from build123d import *

# Parameters (mm, degrees)
BOSS_EXTRUDE2_DEPTH = 3.175
FILLET3_R           = 7.62
FILLET4_R           = 5.08


with BuildPart() as part:
    # Sketch2 → Boss-Extrude2 (new body)
    with BuildSketch(Plane(origin=(0, 0, 0), x_dir=(1, 0, 0), z_dir=(0, 1, 0))):
        Polygon((444.5, 96.52), (0, 96.52), (57.15, 0), (444.5, 0), align=None)
    extrude(amount=BOSS_EXTRUDE2_DEPTH)

    # Fillet3
    fillet3_edges = [part.edges().sort_by_distance(p)[0] for p in [
        (57.15, 1.5875, 0),
        (444.5, 1.5875, -96.52),
        (444.5, 1.5875, 0),
    ]]
    fillet(fillet3_edges, radius=FILLET3_R)

    # Fillet4
    fillet4_edges = [part.edges().sort_by_distance(p)[0] for p in [
        (0, 1.5875, -96.52),
    ]]
    fillet(fillet4_edges, radius=FILLET4_R)


solid = part.part
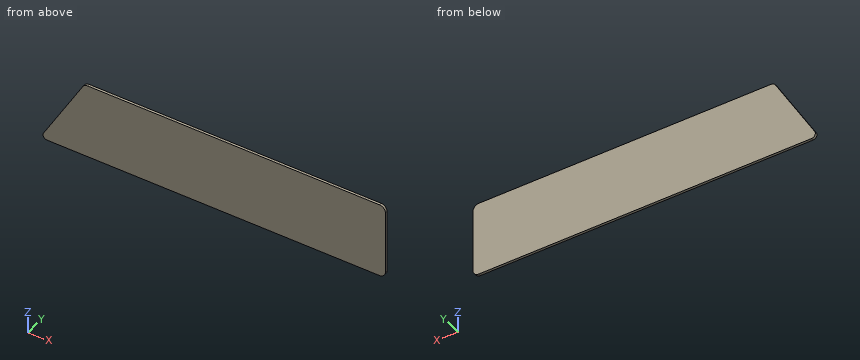
Source: CAD feature listing. Evaluate the final solid. Frame: model axes, mm. Coordinates: 2 decimals unless noted, no trailing zeros. Loops run counter-clockwise (first coordinate to the right, second up) from the corner with the lowest first, then second, coordinate; pieces in that order, holes last. Notation, with made-up numbers: (21.25, 10) - (68.25, 10) arc R17 cw to (68.25, 23) - close; hole circle Ø2 at (76.25, 66). An arc over 180 degrees is marked (long way). One line per question, with ' | ' between items.
1) Section C-C, the plane z = -45.5. Return loops of the section in (x, y) (3 decimals).
Report:
outline: (30.209, 0) - (444.5, 0) - (444.5, 3.175) - (30.209, 3.175) - close
2) Line query: line 1 along Z through (x, y) = (42.5, 0.8); line 2 along X through (y, z) = (0.8, -14.5); line 3 along X through (y, z) = (1.75, -70). Output: solid intervals per line, ascending.
Report:
line 1: z = -96.52 to -24.74 | line 2: x = 48.56 to 444.5 | line 3: x = 15.7 to 444.5
3) First-contact query: P1, Ø1, axis at y = 1.5, z = -66.5, coming from the -X side. Flat tip, straight axial feed; report the tip coordinate or a pass-through.
Report:
P1: stops at x = 17.48
4) Section A-A, the plane y = 2.45. Return loops of the section in (x, z), then the cut area to 3 significant figures.
Report:
outline: (4.54, -88.85) arc R5.08 ccw to (8.91, -96.52) - (436.88, -96.52) arc R7.62 ccw to (444.5, -88.9) - (444.5, -7.62) arc R7.62 ccw to (436.88, 0) - (61.49, 0) arc R7.62 ccw to (54.94, -3.74) - close | area: 40,100 mm²
5) Section B-B, the plane z = -19. Return loops of the section in (x, y) (3 decimals), then the cut area to 3 significant figures.
Report:
outline: (45.9, 0) - (444.5, 0) - (444.5, 3.175) - (45.9, 3.175) - close | area: 1,270 mm²
